Geometry check sheet. Reference: the model listing, model coordinates, mm. Face numbers are marked on the shaded views. A direction names the side the tool comes from. Coordinates: 2 decimals unless noted, no trailing zeros. Loops run counter-clockwise (first coordinate to the right, second up) from the corner with the lowest first, then second, coordinate; pieces in that order, holes last.
from build123d import *

# Parameters (mm, degrees)
SKETCH2_R           = 7
BOSS_EXTRUDE1_DEPTH = 25
SKETCH3_R           = 7
BOSS_EXTRUDE2_DEPTH = 17
BOSS_EXTRUDE2_TAPER = 4.289
SKETCH4_R           = 5
BOSS_EXTRUDE3_DEPTH = 18
CHAMFER1_SIZE       = 2
SKETCH5_R           = 12.5
BOSS_EXTRUDE4_DEPTH = 4


with BuildPart() as part:
    # Sketch2 → Boss-Extrude1 (new body)
    with BuildSketch(Plane(origin=(0, 0, 0), x_dir=(1, 0, 0), z_dir=(0, 1, 0))):
        with Locations(Location((0, 0, 0), (0, 0, 270))):
            Circle(SKETCH2_R)
    extrude(amount=BOSS_EXTRUDE1_DEPTH)

    # Sketch3 → Boss-Extrude2 (add)
    with BuildSketch(Plane(origin=(0, 25, 0), x_dir=(1, 0, 0), z_dir=(0, 1, 0))):
        with Locations(Location((0, 0, 0), (0, 0, 270))):
            Circle(SKETCH3_R)
    extrude(amount=BOSS_EXTRUDE2_DEPTH, taper=BOSS_EXTRUDE2_TAPER)

    # Sketch4 → Boss-Extrude3 (add)
    with BuildSketch(Plane(origin=(0, 42, 0), x_dir=(1, 0, 0), z_dir=(0, 1, 0))):
        with Locations(Location((0, 0, 0), (0, 0, 270))):
            Circle(SKETCH4_R)
    extrude(amount=BOSS_EXTRUDE3_DEPTH)

    # Chamfer1
    chamfer1_edges = [part.edges().sort_by_distance(p)[0] for p in [
        (0, 60, -5),
    ]]
    chamfer(chamfer1_edges, length=CHAMFER1_SIZE)

    # Sketch5 → Boss-Extrude4 (add)
    with BuildSketch(Plane.XZ):
        with Locations(Location((0, 0, 0), (0, 0, 270))):
            Circle(SKETCH5_R)
    extrude(amount=BOSS_EXTRUDE4_DEPTH)


solid = part.part
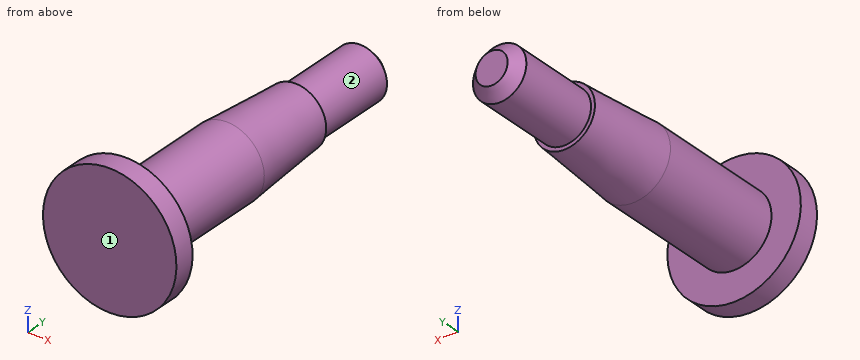
(1) Gauge pin test, flat ends, axial feed: pin 1 Ø8 at (x, z) = (6.5, 3) entering from +Y; pin 2 Ø8 at (y, z) = (41, -7) entering from +X; pin 3 Ø8 at (x, z) = (3, 7.5) entering from +Y. Record the tip position at first contact, or that the pin passes through.
Findings:
pin 1: stops at y = 59.84
pin 2: stops at x = 4.99
pin 3: stops at y = 58.92
(2) Sectioned sample at D-D on z = -9.75. Record the cut outline in (x, y).
Findings:
outline: (-7.82, -4) - (7.82, -4) - (7.82, 0) - (-7.82, 0) - close
(3) Scan lines: L1, parallel to Y at x = -7, z = -2.5; L2, parallel to Z at x = 3, y = 31.5; L3, parallel to Y at x = 0.5, z = 3. Record each from-to range of solid material in increasing order.
Findings:
L1: y = -4 to 0
L2: z = -5.78 to 5.78
L3: y = -4 to 59.96
(4) Sectioned sample at C-C on y = 2.5. Record the cut outline in (x, z).
Findings:
outline: circle Ø14 at (0, 0)
(5) Access from +Z, -Z, +X, -X, +Y, -Y to the whole of each face (thin tool, end or side, straight path). Record for the marked faces 1 and 2.
Findings:
face 1: +Z, -Z, +X, -X, -Y
face 2: +Y
(6) Sectioned sample at B-B on y = 52.5. Record the cut outline in (x, z), and give its area (3 significant figures).
Findings:
outline: circle Ø10 at (0, 0)
area: 78.5 mm2
(7) Sectioned sample at A-A on z = 0. Record the cut outline in (x, y), and give its area (3 significant figures).
Findings:
outline: (-12.5, -4) - (12.5, -4) - (12.5, 0) - (7, 0) - (7, 25) - (5.73, 42) - (5, 42) - (5, 58) - (3, 60) - (-3, 60) - (-5, 58) - (-5, 42) - (-5.73, 42) - (-7, 25) - (-7, 0) - (-12.5, 0) - close
area: 842 mm2
